from build123d import *

# Parameters (mm, degrees)
F0_R     = 3.25
F0_W     = 67
F0_H     = 37
F1_DEPTH = 1.6
F2_W     = 20
F2_H     = 7
F3_DEPTH = 6
F4_W     = 5.5
F4_H     = 15
F5_DEPTH = 3


with BuildPart() as f1:
    # F0 (on Front) → F1 (new body)
    with BuildSketch(Plane.XZ):
        Polygon((-116.5, -30.3), (116.5, -30.3), (116.5, 30.3), (102.9, 30.3), (102.9, 19.57), (96.1, 19.57), (96.1, 30.3), (86.9, 30.3), (86.9, 19.57), (80.1, 19.57), (80.1, 30.3), (-116.5, 30.3), align=None)
        with Locations((91.5, -6.62)):
            Circle(F0_R, mode=Mode.SUBTRACT)
        with Locations((-63, 1.8)):
            Rectangle(F0_W, F0_H, mode=Mode.SUBTRACT)
    extrude(amount=F1_DEPTH)

    # F2 (on face) → F3 (join)
    with BuildSketch(Plane(origin=(0, 0, 0), x_dir=(-1, 0, 0), z_dir=(0, 1, 0))):
        with Locations((21.5, -21.8)):
            Rectangle(F2_W, F2_H)
    extrude(amount=F3_DEPTH)

    # F4 (on face) → F5 (join)
    with BuildSketch(Plane(origin=(0, 0, 0), x_dir=(-1, 0, 0), z_dir=(0, 1, 0))):
        with Locations((100.25, 20.8)):
            Rectangle(F4_W, F4_H)
    extrude(amount=F5_DEPTH)


solid = f1.part
Geometry: final body of the model. Coordinates: model frame, mm. A direction names the side the tool comes from. Round coordinates to 2 decimals unless told otherwise and drop trailing zeros. Order: outer loops, then holes, each group sorted by start corner. A loop starts at its lowest first (then second) coordinate and runs counter-clockwise, first axis right, second up.
Q1. Material intervals for probe 1 along Z at (x, y) = (91.5, -0.9); probe 2 along Z at (x, y) = (-53, -0.5); probe 3 along Y at (x, z) = (18, 18.5), sorted ascending.
Result sheet:
probe 1: z = -30.3 to -9.87, -3.37 to 30.3
probe 2: z = -30.3 to -16.7, 20.3 to 30.3
probe 3: y = -1.6 to 0
Q2. Section B-B, the plane x = 91.5. Output: boundary loops of the cut face in (y, z), and give its area (3 significant figures).
Result sheet:
outline: (-1.6, -30.3) - (0, -30.3) - (0, -9.87) - (-1.6, -9.87) - close; (-1.6, -3.37) - (0, -3.37) - (0, 30.3) - (-1.6, 30.3) - close
area: 86.6 mm2
Q3. Pin query (flat end, axial travel): pin 1 (6 mm diameter, centred on x = 7.5, z = 13.5, fed in from +Y); pin 2 (3.5 mm diameter, centred on y = 2, z = 17.5, fed in from +X); pin 3 (3 mm diameter, centred on x = -14.5, y = 4, fed in from -Z). Return the tip coordinate at first contact, or that it passes through.
Result sheet:
pin 1: stops at y = 0
pin 2: stops at x = -97.5
pin 3: stops at z = -25.3
Q4. Mould query, pull axis Z, two halves, no side actions, for faces 1 (the face through (-21, 3, -18.3)), 2 (the face through (88.253, -0.789, -6.477)), 3 (the face through (-21, 6, -22)). Classes: released by +Z, released by -Z, zero draft, split by the parting line, or undercut.
Result sheet:
face 1: released by +Z
face 2: undercut
face 3: zero draft
Q5. Section A-A, the plane z = 1. Output: boundary loops of the cut face in (x, y).
Result sheet:
outline: (-116.5, -1.6) - (-96.5, -1.6) - (-96.5, 0) - (-116.5, 0) - close; (-29.5, -1.6) - (116.5, -1.6) - (116.5, 0) - (-29.5, 0) - close
Q6. Section C-C, the plane y = 4.25. Output: boundary loops of the cut face in (x, z).
Result sheet:
outline: (-31.5, -25.3) - (-11.5, -25.3) - (-11.5, -18.3) - (-31.5, -18.3) - close
Q7. Section D-D, the plane x = 42. Output: boundary loops of the cut face in (y, z).
Result sheet:
outline: (-1.6, -30.3) - (0, -30.3) - (0, 30.3) - (-1.6, 30.3) - close
Q8. Access query for faces 4 (the face through (-31.5, 3, -22)), 5 (the face through (-21, 3, -25.3)), 6 (the face through (-11.5, 3, -22)). Directions: +Z, -Z, +X, -X, +Y, -Y. A direction counts if a zero-diameter tool reaches every point of the face in a straight line with its end or side. Return the directions, or none.
Result sheet:
face 4: +Z, -Z, -X, +Y
face 5: -Z, +X, -X, +Y
face 6: +Z, -Z, +X, +Y
